from build123d import *

# Parameters (mm, degrees)
BOSS_EXTRUDE1_DEPTH      = 60
SKETCH25_W               = 5.5
SKETCH25_H               = 17
BOSS_EXTRUDE3_DEPTH      = 20
FILLET1_R                = 2.3
CUT_EXTRUDE19_DEPTH      = 165.638713704
CUT_EXTRUDE19_DEPTH_BACK = 165.638713704
SKETCH30_W               = 183.61
SKETCH30_H               = 30
SKETCH31_R               = 4
CUT_EXTRUDE20_DEPTH      = 220.90493429


with BuildPart() as part:
    # Sketch1 → Boss-Extrude1 (new body)
    with BuildSketch(Plane(origin=(0, 0, 0), x_dir=(1, 0, 0), z_dir=(0, 1, 0))):
        with BuildLine():
            Line((91.805, -10), (90.252689849, -10))
            ThreePointArc((90.252689849, -10), (0, -90.805), (-90.252689849, -10))
            Line((-90.252689849, -10), (-91.805, -10))
            Line((-91.805, -10), (-91.805, 20))
            Line((-91.805, 20), (-76.805, 20))
            Line((-76.805, 20), (-76.805, 0))
            ThreePointArc((-76.805, 0), (0, -76.805), (76.805, 0))
            Line((76.805, 0), (76.805, 20))
            Line((76.805, 20), (91.805, 20))
            Line((91.805, 20), (91.805, -10))
        make_face()
    extrude(amount=-BOSS_EXTRUDE1_DEPTH)

    # Sketch25 → Boss-Extrude3 (add)
    with BuildSketch(Plane(origin=(0, -60, 0), x_dir=(-1, 0, 0), z_dir=(0, -1, 0))):
        with Locations((84.305, 5)):
            Rectangle(SKETCH25_W, SKETCH25_H)
        with Locations((-84.305, 5)):
            Rectangle(SKETCH25_W, SKETCH25_H)
    extrude(amount=BOSS_EXTRUDE3_DEPTH)

    # Fillet1
    fillet1_edges = [part.edges().sort_by_distance(p)[0] for p in [
        (84.305, -60, 3.5),
        (81.555, -60, -5),
        (87.055, -60, -5),
        (84.305, -60, -13.5),
        (-84.305, -60, 3.5),
        (-87.055, -60, -5),
        (-81.555, -60, -5),
        (-84.305, -60, -13.5),
    ]]
    fillet(fillet1_edges, radius=FILLET1_R)

    # Sketch30 → Cut-Extrude19 (cut, two sides: drawn at the far end of the back side and taken through both)
    with BuildSketch(Plane(origin=(0, 0, -20), x_dir=(-1, 0, 0), z_dir=(0, 0, -1)).offset(-CUT_EXTRUDE19_DEPTH_BACK)):
        with Locations((0, -15)):
            Rectangle(SKETCH30_W, SKETCH30_H)
    extrude(amount=CUT_EXTRUDE19_DEPTH + CUT_EXTRUDE19_DEPTH_BACK, mode=Mode.SUBTRACT)

    # Sketch31 → Cut-Extrude20 (cut, through all)
    with BuildSketch(Plane(origin=(91.805, 0, 0), x_dir=(0, 0, -1), z_dir=(1, 0, 0))):
        with Locations((7, -45)):
            Circle(SKETCH31_R)
    extrude(amount=-CUT_EXTRUDE20_DEPTH, mode=Mode.SUBTRACT)


solid = part.part
Read the model definition and answer for the solid it produces. Units are mm, in the model's axes. A direction names the side the tool comes from. Round coordinates to 2 decimals unless told otherwise and drop trailing zeros. Write each loop counter-clockwise with the first axis right and the second up, starting at its lowest first coordinate (ties: lowest second). Pieces come first, ordered by that corner, then holes.
1. The part is cut by section B-B, the plane z = 47. Determine the outline of the cut face in (x, y).
2. Which of the six approach directions +Z, -Z, +X, -X, +Y, -Y give full straight-line access (tool end or side, diameter ignored) to faces 4 (the face through (81.555, -71, -5)), 5 (the face through (-84, -71, 3.5)), 6 (the face through (76.805, -45, -12)), 7 (the face through (87.055, -71, -5))?
3. The part is cut by section D-D, the plane y = -35.5. Determine the outline of the cut face in (x, z) (3 decimals).
4. The part is cut by section A-A, the plane y = -45. Determine the outline of the cut face in (x, z) (3 decimals), then the cut area to 3 significant figures.
5. Determine the mould class of faces 1 (the face through (-6, -30, 77)), 2 (the face through (-84.2, -41.034, -6.479)), 3 (the face through (84, -71, -13.5)) for opening direction Y: pulls with the +Y half, pulls with the -Y half, needs draft (parallel to the pull), parting line crosses it, or undercut.
6. The part is cut by section C-C, the plane z = -7. Determine the outline of the cut face in (x, y) (3 decimals).
7. Given pin 1 Ø7 at (y, z) = (-45, -7) entering from -X; pin 2 Ø8.5 at (y, z) = (-71.5, -3.5) entering from -X (3 decimals); pin 3 Ø4.5 at (x, y) = (85, -72.5) entering from +Z; pin 4 Ø8 at (y, z) = (-38, 79) entering from -X, each flat-ended and moving along its own axis, determine where each tip first touches the part or whether it passes through.
8. Straight lines are drawn through the part: L1, parallel to Y at x = -86, z = -7; L2, parallel to X at y = -34, z = -10 (3 decimals); L3, parallel to Y at x = -80.5, z = -7. For each, find the intervals that lie inside material, in ascending order.
Values:
1. outline: (-77.7, -60) - (-60.75, -60) - (-60.75, -30) - (-77.7, -30) - close; (60.75, -60) - (77.7, -60) - (77.7, -30) - (60.75, -30) - close
2. face 4: +Z, -Z, -Y
2. face 5: +Z, +X, -X, -Y
2. face 6: -Z, +Y, -Y
2. face 7: +Z, -Z, +X, -Y
3. outline: (-91.805, -20) - (-76.805, -20) - (-76.805, 0) arc R76.805 cw to (76.805, 0) - (76.805, -20) - (91.805, -20) - (91.805, 10) - (90.253, 10) arc R90.805 ccw to (-90.253, 10) - (-91.805, 10) - close
4. outline: (-91.805, -20) - (-76.805, -20) - (-76.805, -11) - (-91.805, -11) - close; (-91.805, -3) - (-76.805, -3) - (-76.805, 0) arc R76.805 cw to (76.805, 0) - (76.805, -3) - (91.805, -3) - (91.805, 10) - (90.253, 10) arc R90.805 ccw to (-90.253, 10) - (-91.805, 10) - close; (76.805, -20) - (91.805, -20) - (91.805, -11) - (76.805, -11) - close
4. area: 4,070 mm2
5. face 1: pulls with the +Y half
5. face 2: undercut
5. face 3: needs draft
6. outline: (-91.805, -60) - (-89.355, -60) arc R2.3 cw to (-87.055, -62.3) - (-87.055, -80) - (-81.555, -80) - (-81.555, -62.3) arc R2.3 cw to (-79.255, -60) - (-76.805, -60) - (-76.805, -49) - (-91.805, -49) - close; (-91.805, -41) - (-76.805, -41) - (-76.805, -30) - (-91.805, -30) - close; (76.805, -60) - (79.255, -60) arc R2.3 cw to (81.555, -62.3) - (81.555, -80) - (87.055, -80) - (87.055, -62.3) arc R2.3 cw to (89.355, -60) - (91.805, -60) - (91.805, -49) - (76.805, -49) - close; (76.805, -41) - (91.805, -41) - (91.805, -30) - (76.805, -30) - close
7. pin 1: passes through
7. pin 2: stops at x = -87.055
7. pin 3: stops at z = 3.5
7. pin 4: stops at x = -51.19
8. L1: y = -80 to -49, -41 to -30
8. L2: x = -91.805 to -76.805, 76.805 to 91.805
8. L3: y = -60.37 to -49, -41 to -30
